from build123d import *

# Parameters (mm, degrees)
BOSS_EXTRUDE1_DEPTH                        = 100
SKETCH2_W                                  = 3
SKETCH2_H                                  = 8
BOSS_EXTRUDE2_DEPTH                        = 8
MIRROR1_AT_THE_SECOND_PLANE_COPY_1_SKETC_W = 3
MIRROR1_AT_THE_SECOND_PLANE_COPY_1_SKETC_H = 8
MIRROR1_AT_THE_SECOND_PLANE_COPY_1_DEPTH   = 8
SKETCH3_R                                  = 1.4
CUT_EXTRUDE1_DEPTH                         = 134.54400024
FILLET1_START                              = -46
FILLET1_DEPTH                              = 47


with BuildPart() as part:
    # Sketch1 → Boss-Extrude1 (new body)
    with BuildSketch(Plane.XY):
        Polygon((-3, 80), (0, 80), (0, 0), (-45, 0), (-45, 77), (-42, 77), (-42, 3), (-3, 3), align=None)
    extrude(amount=BOSS_EXTRUDE1_DEPTH)

    # Sketch2 → Boss-Extrude2 (add)
    with BuildSketch(Plane(origin=(-42, 0, 0), x_dir=(0, 0, -1), z_dir=(1, 0, 0))):
        with Locations((-95.5, 7)):
            Rectangle(SKETCH2_W, SKETCH2_H)
    boss_extrude2 = extrude(amount=BOSS_EXTRUDE2_DEPTH)

    # Mirror1: Boss-Extrude2 across plane
    add(boss_extrude2.mirror(Plane.ZX.offset(36)))

    # Mirror1 at the second plane: Boss-Extrude2 across plane
    add(boss_extrude2.mirror(Plane.XY.offset(50)))

    # Mirror1 at the second plane copy 1 sketc → Mirror1 at the second plane copy 1 (add)
    with BuildSketch(Plane(origin=(-42, 72, 100), x_dir=(0, 0, 1), z_dir=(1, 0, 0))):
        with Locations((-95.5, 7)):
            Rectangle(MIRROR1_AT_THE_SECOND_PLANE_COPY_1_SKETC_W, MIRROR1_AT_THE_SECOND_PLANE_COPY_1_SKETC_H)
    extrude(amount=MIRROR1_AT_THE_SECOND_PLANE_COPY_1_DEPTH)

    # Sketch3 → Cut-Extrude1 (cut, through all)
    with BuildSketch(Plane.XY.offset(97)):
        with Locations((-38, 7)):
            Circle(SKETCH3_R)
    cut_extrude1 = extrude(amount=-CUT_EXTRUDE1_DEPTH, mode=Mode.SUBTRACT)

    # Mirror2: Cut-Extrude1 across plane
    add(cut_extrude1.mirror(Plane.ZX.offset(36)), mode=Mode.SUBTRACT)

    # Fillet1: read off the stored shape, not the designer's step
    # Fillet1 outline → Fillet1 (cut)
    with BuildSketch(Plane.YZ.offset(FILLET1_START)):
        with BuildLine():
            Line((80, 0), (80, 3))
            ThreePointArc((80, 3), (79.121320344, 0.878679656), (77, 0))
            Line((77, 0), (80, 0))
        make_face()
        with BuildLine():
            ThreePointArc((77, 100), (79.121320344, 99.121320344), (80, 97))
            Line((80, 97), (80, 100))
            Line((80, 100), (77, 100))
        make_face()
        with BuildLine():
            Line((0, 0), (3, 0))
            ThreePointArc((3, 0), (0.878679656, 0.878679656), (0, 3))
            Line((0, 3), (0, 0))
        make_face()
        with BuildLine():
            ThreePointArc((0, 97), (0.878679656, 99.121320344), (3, 100))
            Line((3, 100), (0, 100))
            Line((0, 100), (0, 97))
        make_face()
    extrude(amount=FILLET1_DEPTH, mode=Mode.SUBTRACT)


solid = part.part
Can you work these out from the model? Positions are in its coordinate system, mm. A direction names the side the tool comes from. Coordinates: 2 decimals unless noted, no trailing zeros. Write each loop counter-clockwise with the first axis right and the second up, starting at its lowest first coordinate (ties: lowest second). Pieces come first, ordered by that corner, then holes. Notation, with made-up numbers: (44, 43) -> (50, 43) arc R6 cw to (50, 52) -> close; hole circle Ø4 at (18.25, 20). An arc over 180 degrees is marked (long way). Write each question's results on one line, items separated by ' | '. Start each with the question number.
Q1. We'd pull the mould along X, two halves only. Please class faces 1 (the face through (-38, 61, 4)), 2 (the face through (-2, 80, 49)), 3 (the face through (-45, 38, 49)): +X half, -X half, draft (parallel to the pull), parting line (faces both ways), or undercut.
Q2. Imagine slicing it at C-C (x = -38). State how many separate pieces and enclosed holes the cut face has, then the cut area to 3 significant figures.
Q3. Imagine slicing it at B-B (y = 19). Write out the boundary of the cut face in (x, z).
Q4. If I drill on probe 1 along X at (y, z) = (65, 3.8); probe 2 along Y at (x, z) = (-38, 5.05); probe 3 along X at (y, z) = (75, 37), over which ranges is the centre line in solid material (lowest first)?
Q5. On a 3-axis mill with a long thin cutter (end or side, diameter ignored), from which of +Z, -Z, +X, -X, +Y, -Y can I reach the whole of each face in a straight line? I mean faces 4 (the face through (-38, 67, 94)), 5 (the face through (-34, 65, 4)), 6 (the face through (-38, 61, 96)), 7 (the face through (-36, 7, 97)), 8 (the face through (-38, 67, 3)). Say none if no direction works.
Q6. I'm going to push flat-ended pins straight in: pin 1 (4 mm diameter, centred on x = -12.5, z = 48, fed in from +Y); pin 2 (5 mm diameter, centred on y = 24, z = 82, fed in from +X); pin 3 (4.5 mm diameter, centred on x = -38, y = 7, fed in from +Z); pin 4 (0.9 mm diameter, centred on x = -43.5, z = 64, fed in from +Y). Where does each tip first touch, or does it pass through?
Q7. Imagine slicing it at D-D (z = 11). Write out the boundary of the cut face in (x, y).
Q8. Imagine slicing it at A-A (y = 65). Write out the boundary of the cut face in (x, z).
Taken from the geometry:
1) face 1: undercut | face 2: draft | face 3: -X half
2) separate pieces: 7 | enclosed holes: 0 | area: 359 mm^2
3) outline: (-45, 0) -> (-42, 0) -> (-42, 100) -> (-45, 100) -> close; (-3, 0) -> (0, 0) -> (0, 100) -> (-3, 100) -> close
4) probe 1: x = -45 to -39.4, -36.6 to -34, -3 to 0 | probe 2: y = 0 to 5.6, 8.4 to 11, 61 to 63.6, 66.4 to 69 | probe 3: x = -45 to -42, -3 to 0
5) face 4: +Y | face 5: +Z, -Z, +Y | face 6: +Z, -Z | face 7: +Z, +Y | face 8: -Z, +Y
6) pin 1: stops at y = 3 | pin 2: stops at x = 0 | pin 3: stops at z = 97 | pin 4: stops at y = 77
7) outline: (-45, 0) -> (0, 0) -> (0, 80) -> (-3, 80) -> (-3, 3) -> (-42, 3) -> (-42, 77) -> (-45, 77) -> close
8) outline: (-45, 0) -> (-42, 0) -> (-42, 3) -> (-39.4, 3) -> (-39.4, 6) -> (-42, 6) -> (-42, 94) -> (-39.4, 94) -> (-39.4, 97) -> (-42, 97) -> (-42, 100) -> (-45, 100) -> close; (-36.6, 3) -> (-34, 3) -> (-34, 6) -> (-36.6, 6) -> close; (-36.6, 94) -> (-34, 94) -> (-34, 97) -> (-36.6, 97) -> close; (-3, 0) -> (0, 0) -> (0, 100) -> (-3, 100) -> close
